```python
from build123d import *

# Parameters (mm, degrees)
SKETCH1_W               = 20
SKETCH1_H               = 10
BOSS_EXTRUDE1_DEPTH     = 20
CUT_EXTRUDE1_DEPTH      = 23.912878475
CUT_EXTRUDE1_DEPTH_BACK = 13


with BuildPart() as part:
    # Sketch1 → Boss-Extrude1 (new body)
    with BuildSketch(Plane.XY):
        Rectangle(SKETCH1_W, SKETCH1_H)
    extrude(amount=BOSS_EXTRUDE1_DEPTH)

    # Sketch2 → Cut-Extrude1 (cut, two sides: drawn at the far end of the back side and taken through both)
    with BuildSketch(Plane.XY.offset(20).offset(-CUT_EXTRUDE1_DEPTH_BACK)):
        Polygon((-6.5, 53.587562763), (-6.5, 5), (-6.5, 1.1), (-7.5, 1.1), (-7.5, 0), (0, 0), (7.5, 0), (7.5, 1.1), (6.5, 1.1), (6.5, 5), (6.5, 53.587562763), (6.5, 150.762688289), (-6.5, 150.762688289), align=None)
    extrude(amount=CUT_EXTRUDE1_DEPTH + CUT_EXTRUDE1_DEPTH_BACK, mode=Mode.SUBTRACT)


solid = part.part
```
Geometry: final body of the model. Coordinates: model frame, mm. A direction names the side the tool comes from. Give positions to 0.01 mm unless a question says otherwise; leave off trailing zeros. Order: outer loops, then holes, each group sorted by start corner. A loop starts at its lowest first (then second) coordinate and runs counter-clockwise, first axis right, second up. Notation, with made-up numbers: (39.5, -31.75) -> (68.5, -31.75) arc R19 cw to (68.5, -8.75) -> close; hole circle Ø2 at (35, 35.25). An arc over 180 degrees is marked (long way). Write each question's results on one line, items separated by ' | '. Start each with the question number.
1) Section D-D (x = 0.75). Return loops of the section in (y, z), then the cut area to 3 significant figures.
2) First-contact query: pin 1 (1.5 mm diameter, centred on x = -3, y = 1.5, fed in from +Z); pin 2 (12 mm diameter, centred on x = -2, z = 11.5, fed in from +Y); pin 3 (6.5 mm diameter, centred on x = -1, z = 10.5, fed in from +Y). Flat tips, straight axial feed; report the tip coordinate or a pass-through.
3) Set-up query: faces 1 (the flat face through (6.5, 3, 13)), 2 (the flat face through (-10, 0, 10)), 3 (the flat face through (-7.5, 0.6, 13.4)). Return all of +Z, -Z, +X, -X, +Y, -Y with unobstructed straight access to the full face (end or side cutting, diameter ignored); none if empty.
4) Section C-C (x = -7.25). Return loops of the section in (y, z).
5) Section B-B (z = 16.5). Return loops of the section in (x, y).
6) Section A-A (y = 0.25). Return loops of the section in (x, z).
7) Line query: line 1 (X direction, y = 2.5, z = 11); line 2 (X direction, y = 1, z = 9.25); line 3 (Z direction, x = -5.5, y = 0.75). Output: solid intervals per line, ascending. Write a range as from..to.
Calculated:
1) outline: (-5, 0) -> (5, 0) -> (5, 7) -> (0, 7) -> (0, 20) -> (-5, 20) -> close | area: 135 mm2
2) pin 1: z = 7 | pin 2: y = 5 | pin 3: y = 0
3) face 1: +Z, +Y | face 2: +Z, -Z, -X, +Y, -Y | face 3: +Z
4) outline: (-5, 0) -> (5, 0) -> (5, 20) -> (1.1, 20) -> (1.1, 7) -> (0, 7) -> (0, 20) -> (-5, 20) -> close
5) outline: (-10, -5) -> (10, -5) -> (10, 5) -> (6.5, 5) -> (6.5, 1.1) -> (7.5, 1.1) -> (7.5, 0) -> (-7.5, 0) -> (-7.5, 1.1) -> (-6.5, 1.1) -> (-6.5, 5) -> (-10, 5) -> close
6) outline: (-10, 0) -> (10, 0) -> (10, 20) -> (7.5, 20) -> (7.5, 7) -> (-7.5, 7) -> (-7.5, 20) -> (-10, 20) -> close
7) line 1: -10..-6.5, 6.5..10 | line 2: -10..-7.5, 7.5..10 | line 3: 0..7
